```python
from build123d import *

# Parameters (mm, degrees)
SKETCH1_W            = 50
SKETCH1_H            = 50
BOSS_EXTRUDE1_DEPTH  = 2
SKETCH2_R            = 1.65
CUT_EXTRUDE1_DEPTH   = 3
LPATTERN1_COUNT      = 5
LPATTERN1_PITCH      = 10
LPATTERN1_COUNT_DIR2 = 5
LPATTERN1_PITCH_DIR2 = 10


with BuildPart() as part:
    # Sketch1 → Boss-Extrude1 (new body)
    with BuildSketch(Plane.XY):
        Rectangle(SKETCH1_W, SKETCH1_H)
    extrude(amount=BOSS_EXTRUDE1_DEPTH)

    # Sketch2 → Cut-Extrude1 (cut, through all)
    with BuildSketch(Plane.XY.offset(2)):
        with Locations((-20, 20)):
            Circle(SKETCH2_R)
    cut_extrude1 = extrude(amount=-CUT_EXTRUDE1_DEPTH, mode=Mode.SUBTRACT)

    # LPattern1: Cut-Extrude1 5 × 5
    with Locations(*[(j * LPATTERN1_PITCH_DIR2, -i * LPATTERN1_PITCH, 0) for i in range(LPATTERN1_COUNT) for j in range(LPATTERN1_COUNT_DIR2) if (i, j) != (0, 0)]):
        add(cut_extrude1, mode=Mode.SUBTRACT)


solid = part.part
```
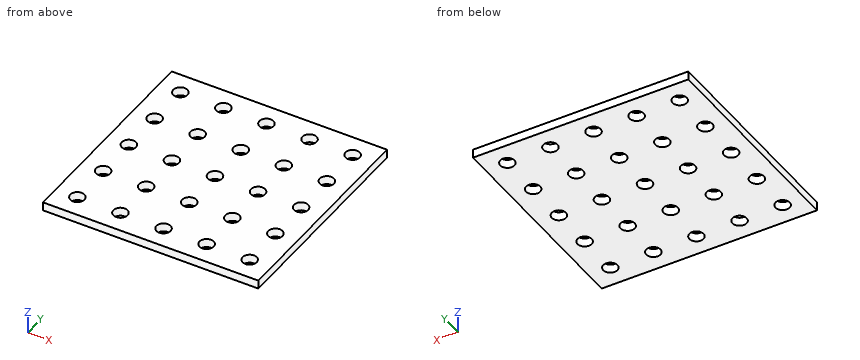
Could you check a few things on this model? Use its own coordinates, in mm. Coordinates: 2 decimals unless noted, no trailing zeros. Write each loop counter-clockwise with the first axis right and the second up, starting at its lowest first coordinate (ties: lowest second). Pieces come first, ordered by that corner, then holes. Notation, with made-up numbers: (61, 72) - (118, 72) arc R23 ccw to (118, 110) - close; hole circle Ø2 at (85.5, -6). An arc over 180 degrees is marked (long way). Use a Markdown table: item, result.
Q1. Imagine slicing it at A-A (x = 10). List the corners of the cut face in (y, z) for me, and give its area (3 significant figures).
Geometry check:
| item | result |
|---|---|
| outline | (-25, 0) - (-21.65, 0) - (-21.65, 2) - (-25, 2) - close; (-18.35, 0) - (-11.65, 0) - (-11.65, 2) - (-18.35, 2) - close; (-8.35, 0) - (-1.65, 0) - (-1.65, 2) - (-8.35, 2) - close; (1.65, 0) - (8.35, 0) - (8.35, 2) - (1.65, 2) - close; (11.65, 0) - (18.35, 0) - (18.35, 2) - (11.65, 2) - close; (21.65, 0) - (25, 0) - (25, 2) - (21.65, 2) - close |
| area | 67.0 mm2 |
Q2. Imagine slicing it at C-C (z = 0.75). Count the separate pieces of the cut face and the enclosed holes in it, and give its area (3 significant figures).
Geometry check:
| item | result |
|---|---|
| separate pieces | 1 |
| enclosed holes | 25 |
| area | 2,290 mm2 |
Q3. Please list where these lines run through material, in increasing order: L1, parallel to Y at x = -20, z = 0.45; L2, parallel to X at y = -9, z = 0.85.
Geometry check:
| item | result |
|---|---|
| L1 | y = -25 to -21.65, -18.35 to -11.65, -8.35 to -1.65, 1.65 to 8.35, 11.65 to 18.35, 21.65 to 25 |
| L2 | x = -25 to -21.31, -18.69 to -11.31, -8.69 to -1.31, 1.31 to 8.69, 11.31 to 18.69, 21.31 to 25 |
